Verification items for this drawing (mm, ordinates from the low corner). Coordinates: 2 decimals unless noted, no trailing zeros. Order: outer loops, then holes, each group sorted by start corner. A loop starts at its lowest first (then second) coordinate and runs counter-clockwise, first axis right, second up.
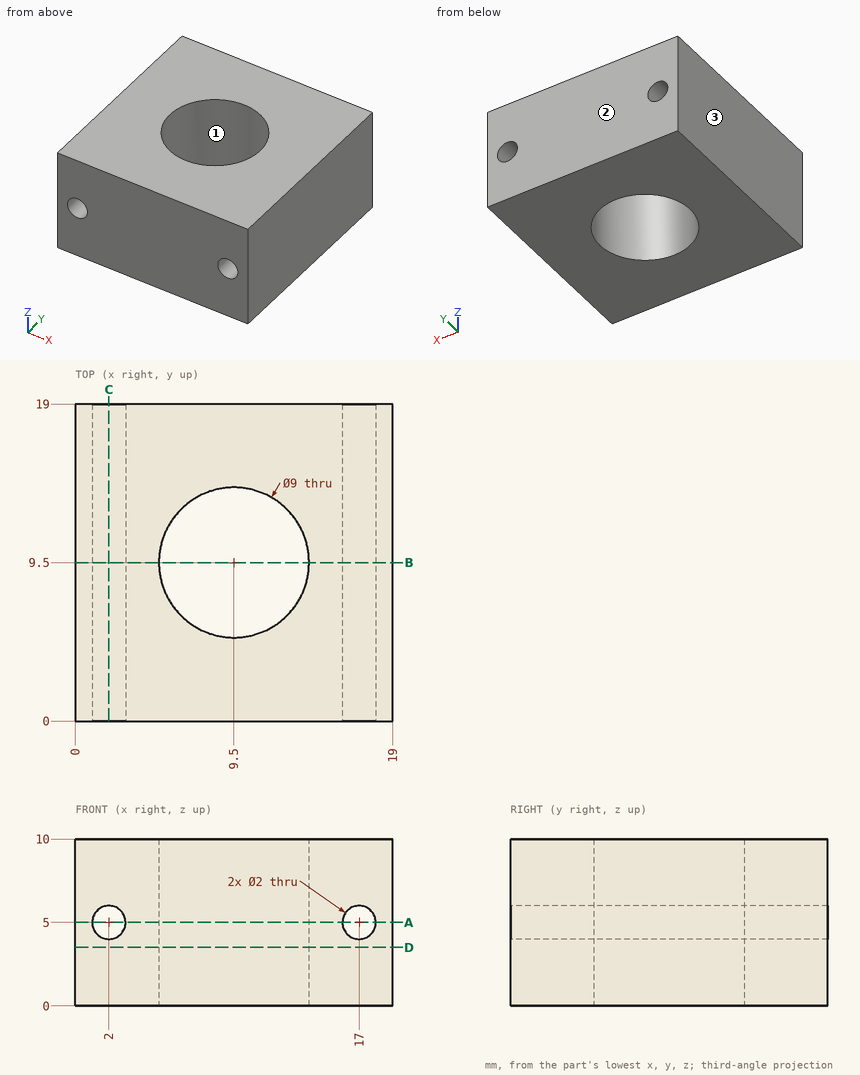
(1) Cross-section at B-B (y = 9.5). Enter the section's corners in (x, z), and give its area (3 significant figures).
Filled in:
outline: (0, 0) - (5, 0) - (5, 10) - (0, 10) - close; (14, 0) - (19, 0) - (19, 10) - (14, 10) - close; hole circle Ø2 at (2, 5); hole circle Ø2 at (17, 5)
area: 93.7 mm2
(2) Thickness scan on probe 1 along Y at (x, z) = (9.5, 2.5); probe 2 along X at (y, z) = (12.5, 5); probe 3 along X at (y, z) = (8, 5). Record the ranges inside material, lowest first.
Filled in:
probe 1: y = 0 to 5, 14 to 19
probe 2: x = 0 to 1, 3 to 6.15, 12.85 to 16, 18 to 19
probe 3: x = 0 to 1, 3 to 5.26, 13.74 to 16, 18 to 19
(3) Cross-section at A-A (z = 5). Enter the section's corners in (x, y), and give its area (3 significant figures).
Filled in:
outline: (0, 0) - (1, 0) - (1, 19) - (0, 19) - close; (3, 0) - (16, 0) - (16, 19) - (3, 19) - close; (18, 0) - (19, 0) - (19, 19) - (18, 19) - close; hole circle Ø9 at (9.5, 9.5)
area: 221 mm2
(4) Cross-section at C-C (x = 2). Enter the section's corners in (y, z).
Filled in:
outline: (0, 0) - (19, 0) - (19, 4) - (0, 4) - close; (0, 6) - (19, 6) - (19, 10) - (0, 10) - close
(5) Release check for a two-part mould opening along Y. For the marked faces 1, 2 and 3 record: +Y half, -Y half, draft (parallel to the pull), parting line (faces both ways), or undercut.
Filled in:
face 1: undercut
face 2: +Y half
face 3: draft
(6) Cross-section at D-D (z = 3.5). Enter the section's corners in (x, y), and give its area (3 significant figures).
Filled in:
outline: (0, 0) - (19, 0) - (19, 19) - (0, 19) - close; hole circle Ø9 at (9.5, 9.5)
area: 297 mm2
